For this review, take the finished solid that the model builds, in its own axes (mm). A direction names the side the tool comes from. Coordinates: 2 decimals unless noted, no trailing zeros. Loops run counter-clockwise (first coordinate to the right, second up) from the corner with the lowest first, then second, coordinate; pieces in that order, holes last.
```python
from build123d import *

# Parameters (mm, degrees)
BOSS_EXTRUDE1_DEPTH                                 = 6.35
CSK_FOR_1_4_FLAT_HEAD_MACHINE_SCREW_100_D           = 6.5278
CSK_FOR_1_4_FLAT_HEAD_MACHINE_SCREW_100_CSINK_D     = 12.8778
CSK_FOR_1_4_FLAT_HEAD_MACHINE_SCREW_100_CSINK_ANGLE = 100
SKETCH5_W                                           = 19.05
SKETCH5_H                                           = 12.7
BOSS_EXTRUDE2_DEPTH                                 = 12.7
BOSS_EXTRUDE3_DEPTH                                 = 12.7


# Read off the part's stored shape, not the designer's step: CBORE for 1/4 Socket Head Cap Screw1
with BuildPart() as part:
    # Sketch1 → Boss-Extrude1 (new body)
    with BuildSketch(Plane.XY):
        with BuildLine():
            Line((0, 0), (0, 88.9))
            ThreePointArc((0, 88.9), (19.05, 107.95), (38.1, 88.9))
            Line((38.1, 88.9), (38.1, 0))
            Line((38.1, 0), (0, 0))
        make_face()
    extrude(amount=-BOSS_EXTRUDE1_DEPTH)

    # CSK for 1/4 Flat Head Machine Screw (100)1 (through all)
    with Locations(Plane.XY):
        with Locations((19.05, 88.9)):
            CounterSinkHole(CSK_FOR_1_4_FLAT_HEAD_MACHINE_SCREW_100_D / 2, CSK_FOR_1_4_FLAT_HEAD_MACHINE_SCREW_100_CSINK_D / 2, counter_sink_angle=CSK_FOR_1_4_FLAT_HEAD_MACHINE_SCREW_100_CSINK_ANGLE)

    # Sketch5 → Boss-Extrude2 (add)
    with BuildSketch(Plane.XY):
        with Locations((19.05, 69.85)):
            Rectangle(SKETCH5_W, SKETCH5_H)
    extrude(amount=BOSS_EXTRUDE2_DEPTH)

    # Sketch6 → Boss-Extrude3 (add)
    with BuildSketch(Plane(origin=(0, 76.2, 0), x_dir=(1, 0, 0), z_dir=(0, 1, 0))):
        with BuildLine():
            Line((9.525, -12.7), (28.575, -12.7))
            ThreePointArc((28.575, -12.7), (19.05, -22.225), (9.525, -12.7))
        make_face()
    extrude(amount=-BOSS_EXTRUDE3_DEPTH)

    # CBORE for 1/4 Socket Head Cap Screw1 out → CBORE for 1/4 Socket Head Cap Screw1 (revolve, cut)
    with BuildSketch(Plane(origin=(19.05, 0, 12.7), x_dir=(1, 0, 0), z_dir=(0, 0, 1))):
        Polygon((0, 63.5), (3.2639, 63.5), (3.2639, 69.85), (5.55625, 69.85), (5.55625, 75.459368711), (6.4389, 76.2), (0, 76.2), align=None)
    revolve(axis=Axis((19.05, 0, 12.7), (0, 1, 0)), mode=Mode.SUBTRACT)

    # Mirror1: part across plane


with BuildPart() as part_1:
    add(part.part)
    add(part.part.mirror(Plane(origin=(38.1, 0, -6.35), x_dir=(0, 0, 1), z_dir=(0, -1, 0))))


solid = part_1.part
```
Q1. Consider section B-B (x = 19.05). Count the separate pieces of the cut face and the enclosed holes in it, then the cut area to 3 significant figures.
Q2. Wall thickness on probe 1 along Y at (x, z) = (19.05, -5.2); probe 2 along X at (y, z) = (67.5, 12.7) (3 decimals); probe 3 along X at (y, z) = (-88.9, -4.1): over which ranges is each line inside the solid? List them lowest first.
Q3. Consider section D-D (x = 32). State the section outline as (y, z) points.
Q4. Consider section C-C (y = 46.5). State the section outline as (x, z) points, then the cut area to 3 significant figures.
Q5. The part is to be moulded in two halves that separate along Y. For faces 1 (the face through (15, -69.85, 13)), 2 (the face through (19.758, 85.714, -4.533)), 3 (the face through (15, 69.85, 13)), say which applies: +Y half, -Y half, draft (parallel to the pull), parting line (faces both ways), or undercut.
Q6. Machinability: for faces 4 (the face through (19, 63.5, 8)), 5 (the face through (19, 76.2, 6)), 6 (the face through (22.037, -72.694, 8.015)), 7 (the face through (28.575, 70, 6)), 8 (the face through (19, -76.2, 6)), which of the approach directions +Z, -Z, +X, -X, +Y, -Y give a long, thin tool a straight path to every point of the face, cutting with its end or side? Answer none if there is none.
Q7. For pin 1 Ø1.5 at (y, z) = (-77, 19) entering from +X; pin 2 Ø10.5 at (x, z) = (19.05, 12.7) entering from +Y; pin 3 Ø5.5 at (x, z) = (18.5, 13.5) entering from -Y; pin 4 Ø5.5 at (x, z) = (20, 6.5) entering from -Y, all flat-tipped, find the tip position at first contact; note any pin that passes through.
Q8. Consider section A-A (z = 2.25). State the section outline as (x, y) points (3 decimals).
Model answer:
1. separate pieces: 5
1. enclosed holes: 0
1. area: 1,610 mm2
2. probe 1: y = -107.95 to -92.16, -85.64 to 85.64, 92.16 to 107.95
2. probe 2: x = 9.525 to 15.786, 22.314 to 28.575
2. probe 3: x = 0 to 15.79, 22.31 to 38.1
3. outline: (-102.87, -6.35) - (102.87, -6.35) - (102.87, 0) - (-102.87, 0) - close
4. outline: (0, -6.35) - (38.1, -6.35) - (38.1, 0) - (0, 0) - close
4. area: 242 mm2
5. face 1: -Y half
5. face 2: undercut
5. face 3: +Y half
6. face 4: +Z, +X, -X
6. face 5: +Z, +X, -X, +Y
6. face 6: -Y
6. face 7: +Z, +X, +Y, -Y
6. face 8: +Z, +X, -X, -Y
7. pin 1: passes through
7. pin 2: stops at y = 69.85
7. pin 3: stops at y = -69.85
7. pin 4: stops at y = -76.2
8. outline: (9.525, -76.2) - (28.575, -76.2) - (28.575, -63.5) - (9.525, -63.5) - close; (9.525, 63.5) - (28.575, 63.5) - (28.575, 76.2) - (9.525, 76.2) - close
